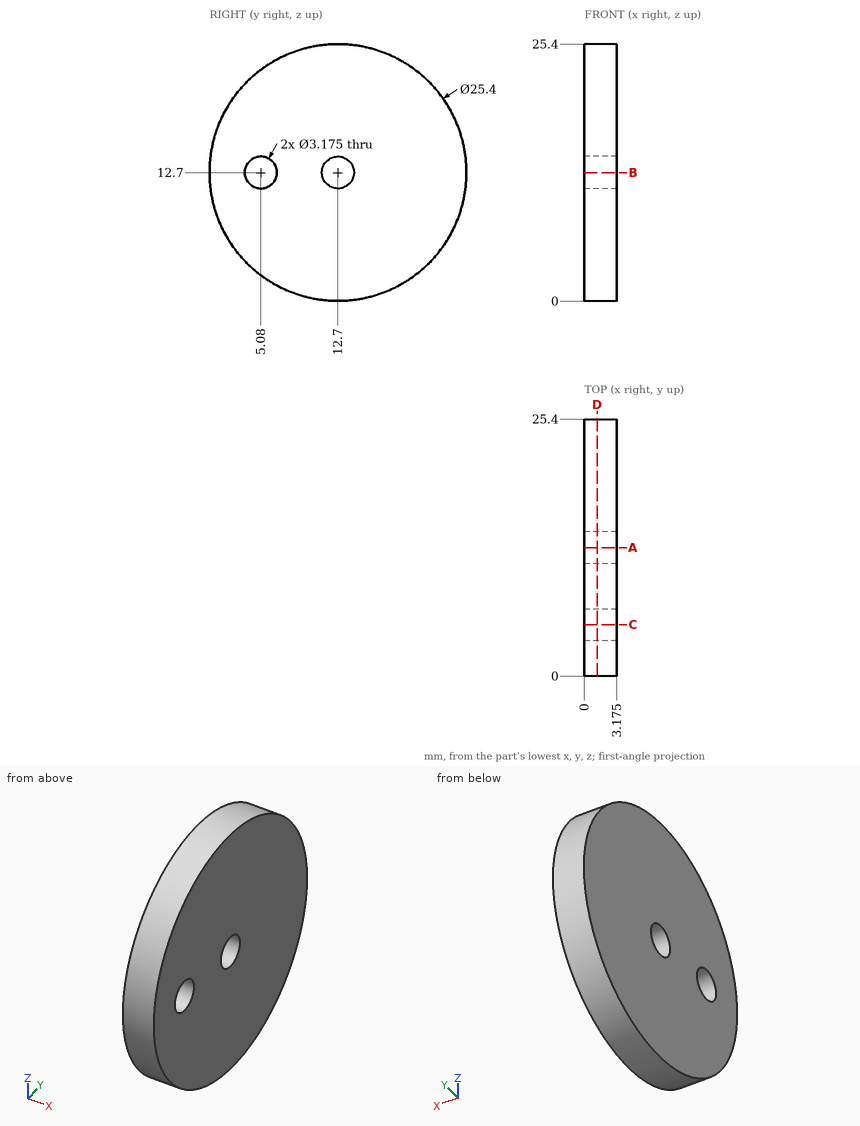
Can you work these out from the drawing? Everything is in mm from the part's minimum corner. Give positions to 0.01 mm unless a question says otherwise; leave off trailing zeros. Loops run counter-clockwise (first coordinate to the right, second up) from the corner with the lowest first, then second, coordinate; pieces in that order, holes last. Notation, with made-up numbers: (0.5, 9.25) -> (33.5, 9.25) arc R13 ccw to (33.5, 20.25) -> close; hole circle Ø8 at (14.25, 57.5). An arc over 180 degrees is marked (long way). Return JSON: item names as keys, results as strings.
Q1. I want a section at C-C, the plane y = 5.08. List the corners of the cut face in (x, z) for me (1 decimal), then the cut area to 3 significant figures.
Checks:
{"outline": "(0, 2.5) -> (3.2, 2.5) -> (3.2, 11.1) -> (0, 11.1) -> close; (0, 14.3) -> (3.2, 14.3) -> (3.2, 22.9) -> (0, 22.9) -> close", "area": "54.4 mm2"}
Q2. I need wall thicknesses on probe 1 along Y at (x, z) = (1.6, 12.7); probe 2 along Y at (x, z) = (1.2, 12); probe 3 along Z at (x, y) = (0.8, 5.08). Which ranges of each line are inside material? Lowest first, please.
Checks:
{"probe 1": "y = 0 to 3.49, 6.67 to 11.11, 14.29 to 25.4", "probe 2": "y = 0.02 to 3.66, 6.5 to 11.28, 14.12 to 25.38", "probe 3": "z = 2.54 to 11.11, 14.29 to 22.86"}
Q3. I want a section at D-D, the plane x = 1.25. List the corners of the cut face in (y, z) for me (1 decimal), then the cut area to 3 significant figures.
Checks:
{"outline": "circle Ø25.4 at (12.7, 12.7); hole circle Ø3.2 at (5.1, 12.7); hole circle Ø3.2 at (12.7, 12.7)", "area": "491 mm2"}
Q4. I want a section at B-B, the plane z = 12.7. List the corners of the cut face in (x, y) for me (1 decimal), then the cut area to 3 significant figures.
Checks:
{"outline": "(0, 0) -> (3.2, 0) -> (3.2, 3.5) -> (0, 3.5) -> close; (0, 6.7) -> (3.2, 6.7) -> (3.2, 11.1) -> (0, 11.1) -> close; (0, 14.3) -> (3.2, 14.3) -> (3.2, 25.4) -> (0, 25.4) -> close", "area": "60.5 mm2"}
Q5. For pin 1 Ø3 at (y, z) = (12.7, 12.7) entering from -X (3 decimals); pin 2 Ø1 at (x, y) = (2, 9.5) entering from -Z, each with a flat end and sliding along its axis, tell me the tip position at first contact or that it passes through.
Checks:
{"pin 1": "passes through", "pin 2": "stops at z = 0.29"}
Q6. I want a section at A-A, the plane y = 12.7. List the corners of the cut face in (x, z) for me (1 decimal).
Checks:
{"outline": "(0, 0) -> (3.2, 0) -> (3.2, 11.1) -> (0, 11.1) -> close; (0, 14.3) -> (3.2, 14.3) -> (3.2, 25.4) -> (0, 25.4) -> close"}
